Model file for the job. Use its own axes, mm. Round coordinates to 2 decimals unless told otherwise and drop trailing zeros. Order: outer loops, then holes, each group sorted by start corner. A loop starts at its lowest first (then second) coordinate and runs counter-clockwise, first axis right, second up. Notation, with made-up numbers: (81, 53.25) - (110, 53.25) arc R20 cw to (110, 88.25) - close; hole circle Ø10 at (-4.75, 32.5). An arc over 180 degrees is marked (long way). Use one line per item in the form item = value.
from build123d import *

# Parameters (mm, degrees)
F0_W     = 3.175
F0_H     = 7.62
F1_DEPTH = 3.175
F3_DEPTH = 3.175
F4_R     = 2.159
F5_DEPTH = 25.4


with BuildPart() as f1:
    # F0 (on Top) → F1 (new body)
    with BuildSketch(Plane.XY):
        with Locations((-1.5875, -3.81)):
            Rectangle(F0_W, F0_H)
    extrude(amount=F1_DEPTH)

    # F2 (on face) → F3 (join)
    with BuildSketch(Plane.YZ):
        with BuildLine():
            Line((-7.62, 3.175), (0, 3.175))
            ThreePointArc((0, 3.175), (-3.81, 6.985), (-7.62, 3.175))
        make_face()
    extrude(amount=-F3_DEPTH)

    # F4 (on face) → F5 (cut)
    with BuildSketch(Plane.YZ):
        with Locations((-3.81, 3.175)):
            Circle(F4_R)
    extrude(amount=-F5_DEPTH, mode=Mode.SUBTRACT)


solid = f1.part
(1) Pull direction Y, two halves, no side cores. Call faces 1 (the face through (-3.175, -6, 5)), 2 (the face through (-2, 0, 2)), 3 (the face through (-1.565, -5.967, 3.27)), 4 (the face through (-2, -7.62, 2)): released by +Y, released by -Y, zero draft, split by the parting line, or undercut.
Report:
face_1 = zero draft
face_2 = released by +Y
face_3 = undercut
face_4 = released by -Y
(2) Slice it at D-D on y = -1. Give the cut face in (x, z) (3 decimals), then the cut area to 3 significant figures.
Report:
outline = (-3.175, 0) - (0, 0) - (0, 5.748) - (-3.175, 5.748) - close
area = 18.2 mm2
(3) Probe probe 1 along Z at (x, y) = (-1.1, -3.81) (3 decimals); probe 2 along Y at (x, z) = (-0.3, 4.75); probe 3 along Y at (x, z) = (-0.9, 2). List the from-to ranges inside material, lowest first. Write a range as [from, to].
Report:
probe_1 = [0, 1.016], [5.334, 6.985]
probe_2 = [-7.28, -5.29], [-2.33, -0.34]
probe_3 = [-7.62, -5.62], [-2, 0]
(4) Slice it at B-B on x = -0.7. Give the cut face in (y, z) (3 decimals).
Report:
outline = (-7.62, 0) - (0, 0) - (0, 3.175) arc R3.81 ccw to (-7.62, 3.175) - close; hole circle Ø4.318 at (-3.81, 3.175)
(5) Slice it at A-A on y = -3.81. Give the cut face in (x, z) (3 decimals).
Report:
outline = (-3.175, 0) - (0, 0) - (0, 1.016) - (-3.175, 1.016) - close; (-3.175, 5.334) - (0, 5.334) - (0, 6.985) - (-3.175, 6.985) - close
(6) Slice it at C-C on z = 4.5. Give the cut face in (x, y) (3 decimals), then the cut area to 3 significant figures.
Report:
outline = (-3.175, -7.382) - (0, -7.382) - (0, -5.515) - (-3.175, -5.515) - close; (-3.175, -2.105) - (0, -2.105) - (0, -0.238) - (-3.175, -0.238) - close
area = 11.9 mm2
